from build123d import *

# Parameters (mm, degrees)
F2_DEPTH = 200
F3_W     = 30
F3_H     = 100
F4_DEPTH = 500
F6_R     = 15
F7_R     = 5


with BuildPart() as f2:
    # F0 (on Front) → F2 (new body)
    with BuildSketch(Plane.XZ):
        with BuildLine():
            Line((-127.5536519289, -36.5021181107), (-127.5536519289, 43.4978818893))
            Line((-127.5536519289, 43.4978818893), (-132.5536519289, 43.4978818893))
            Line((-132.5536519289, 43.4978818893), (-132.5536519289, -36.5021181107))
            ThreePointArc((-132.5536519289, -36.5021181107), (-125.2313214586, -54.1797876403), (-107.5536519289, -61.5021181107))
            Line((-107.5536519289, -61.5021181107), (102.4463480711, -61.5021181107))
            ThreePointArc((102.4463480711, -61.5021181107), (120.1240176008, -54.1797876403), (127.4463480711, -36.5021181107))
            Line((127.4463480711, -36.5021181107), (127.4463480711, 43.4978818893))
            Line((127.4463480711, 43.4978818893), (122.4463480711, 43.4978818893))
            Line((122.4463480711, 43.4978818893), (122.4463480711, -36.5021181107))
            ThreePointArc((122.4463480711, -36.5021181107), (116.5884836948, -50.6442537344), (102.4463480711, -56.5021181107))
            Line((102.4463480711, -56.5021181107), (-107.5536519289, -56.5021181107))
            ThreePointArc((-107.5536519289, -56.5021181107), (-121.6957875526, -50.6442537344), (-127.5536519289, -36.5021181107))
        make_face()
    extrude(amount=F2_DEPTH)


with BuildPart() as f4:
    # F3 (on offset) → F4 (new body)
    with BuildSketch(Plane.YZ.offset(200)):
        with Locations((-145, -29.9103426556)):
            Rectangle(F3_W, F3_H)
    extrude(amount=-F4_DEPTH)


with BuildPart() as f4b:
    # F3 (on offset) → F4, piece 2 (new body)
    with BuildSketch(Plane.YZ.offset(200)):
        with Locations((-35, -29.9103426556)):
            Rectangle(F3_W, F3_H)
    extrude(amount=-F4_DEPTH)


with BuildPart() as f2_1:
    add(f2.part)

    # F5: cut F4, F4b
    add(f4.part, mode=Mode.SUBTRACT)
    add(f4b.part, mode=Mode.SUBTRACT)

    # F6
    f6_edges = [f2_1.edges().sort_by_distance(p)[0] for p in [
        (-130.053652, -200, 43.497882),
        (-130.053652, 0, 43.497882),
        (124.946348, -200, 43.497882),
        (124.946348, 0, 43.497882),
    ]]
    fillet(f6_edges, radius=F6_R)

    # F7
    f7_edges = [f2_1.edges().sort_by_distance(p)[0] for p in [
        (124.946348, -20, 20.089657),
        (124.946348, -50, 20.089657),
    ]]
    fillet(f7_edges, radius=F7_R)


solid = f2_1.part
Can you work these out from the model? Positions are in its coordinate system, mm. A direction names the side the tool comes from. Give positions to 0.01 mm unless a question says otherwise; leave off trailing zeros. Write each loop counter-clockwise with the first axis right and the second up, starting at its lowest first coordinate (ties: lowest second). Pieces come first, ordered by that corner, then holes. Notation, with made-up numbers: (8.5, -31) -> (54.5, -31) arc R26 ccw to (54.5, -15) -> close; hole circle Ø3 at (36.25, 28.25). An arc over 180 degrees is marked (long way). Answer as a JSON object with one key per item and string values. Group by question number.
Item 1: I'm going to push flat-ended pins straight in: P1, Ø1.5, axis at x = 126, y = -149, coming from the -Z side; P2, Ø10, axis at x = 14.5, y = -9, coming from the +Z side. Where does each tip first touch, or does it pass through?
Item 2: Suppose I cut it at D-D (x = 109.5). Please give me the cut outline in (y, z).
Item 3: Please list where these lines run through material, in increasing order: line 1 (X direction, y = -159.5, z = 34); line 2 (Z direction, x = 91, y = -191); line 3 (X direction, y = -81, z = -46.5). Write a range as [from, to].
Item 4: We'd pull the mould along X, two halves only. Please class faces 1 (the face through (119.9, -9.9, -54.4)), 2 (the face through (-132.554, -99, 4)), 3 (the face through (116.74, -89.44, -50.49)): +X half, -X half, draft (parallel to the pull), parting line (faces both ways), or undercut.
Item 5: Suppose I cut it at A-A (x = -48). Please give me the cut outline in (y, z), plus the area to 3 significant figures.
Item 6: Suppose I cut it at B-B (z = -10). Please give me the cut outline in (x, y).
Item 7: For faces 4 (the face through (122.446, -99, 4)), 5 (the face through (-4, -10, -61.502)), 6 (the face through (27, -130, -57)), which set-ups out of +Z, -Z, +X, -X, +Y, -Y let a thin tool reach every point of the face, with its end or its side?
Item 8: Suppose I cut it at C-C (y = -164). Please give me the cut outline in (x, z), plus the area to 3 significant figures.
Findings:
{
 "1": {"P1": "stops at z = 20.09", "P2": "stops at z = -56.5"},
 "2": {"outline": "(-200, -60.49) -> (-160, -60.49) -> (-160, -55.22) -> (-200, -55.22) -> close; (-130, -60.49) -> (-50, -60.49) -> (-50, -55.22) -> (-130, -55.22) -> close; (-20, -60.49) -> (0, -60.49) -> (0, -55.22) -> (-20, -55.22) -> close"},
 "3": {"line 1": "x = [-132.55, -127.55], [122.45, 127.45]", "line 2": "z = [-61.5, -56.5]", "line 3": "x = [-130.47, -124.88], [119.77, 125.36]"},
 "4": {"face 1": "+X half", "face 2": "-X half", "face 3": "undercut"},
 "5": {"outline": "(-200, -61.5) -> (-160, -61.5) -> (-160, -56.5) -> (-200, -56.5) -> close; (-130, -61.5) -> (-50, -61.5) -> (-50, -56.5) -> (-130, -56.5) -> close; (-20, -61.5) -> (0, -61.5) -> (0, -56.5) -> (-20, -56.5) -> close", "area": "700 mm²"},
 "6": {"outline": "(-132.55, -200) -> (-127.55, -200) -> (-127.55, -160) -> (-132.55, -160) -> close; (-132.55, -130) -> (-127.55, -130) -> (-127.55, -50) -> (-132.55, -50) -> close; (-132.55, -20) -> (-127.55, -20) -> (-127.55, 0) -> (-132.55, 0) -> close; (122.45, -200) -> (127.45, -200) -> (127.45, -160) -> (122.45, -160) -> close; (122.45, -130) -> (127.45, -130) -> (127.45, -50) -> (122.45, -50) -> close; (122.45, -20) -> (127.45, -20) -> (127.45, 0) -> (122.45, 0) -> close"},
 "7": {"face 4": "+Z, +Y, -Y", "face 5": "-Z, +X, -X, +Y, -Y", "face 6": "-Z, +X, -X"},
 "8": {"outline": "(-132.55, -36.5) arc R25 ccw to (-107.55, -61.5) -> (102.45, -61.5) arc R25 ccw to (127.45, -36.5) -> (127.45, 43.5) -> (122.45, 43.5) -> (122.45, -36.5) arc R20 cw to (102.45, -56.5) -> (-107.55, -56.5) arc R20 cw to (-127.55, -36.5) -> (-127.55, 43.5) -> (-132.55, 43.5) -> close", "area": "2,200 mm²"}
}
